The listing builds one solid part. Answer for the finished solid, in the listing's coordinates (mm). Face numbers are marked on the shaded views. A direction names the side the tool comes from. Give positions to 0.01 mm unless a question says otherwise; leave off trailing zeros. Loops run counter-clockwise (first coordinate to the right, second up) from the corner with the lowest first, then second, coordinate; pieces in that order, holes last. Notation, with made-up numbers: M 19,48.25 L 24,48.25 A17 ccw 24,69.25 Z; hole C 38.5,73 d7. An arc over 180 degrees is marked long. Use one line per item in the form item = value. Start each with the question number.
1. The mould has two halves that part along X. Classify the marked faces 1, 2 and 3: released by +X, released by -X, zero draft, split by the parting line, or undercut.
2. The part is cut by section C-C (z = 5). Write down the section's boundary in (x, y).
3. Straight lines are drawn through the part: line 1 (Y direction, x = 0, z = 7); line 2 (Z direction, x = 3, y = -2.75); line 3 (X direction, y = 1.25, z = 8.25). For each, find the intervals that lie inside material, in ascending order. Write a range as from..to.
4. For the marked faces 4 and 5, determine the directions among +Z, -Z, +X, -X, +Y, -Y from which every point of the face is accessible in a straight line to the end or side of a thin tool.
5. The part is cut by section A-A (y = 0). Write down the section's boundary in (x, z).
6. Each of these flat-tipped pins is pushed along its axis until it touches: pin 1 Ø3.5 at (x, y) = (0, 0) entering from -Z; pin 2 Ø4 at (x, z) = (-1.5, 6) entering from -Y. Where does it stop, or does it pass through?
Autodesk Inventor part; units mm, degrees
ref_plane "YZ Plane" through (0, 0, 0) normal (1, 0, 0) x (0, 1, 0)
ref_plane "XZ Plane" through (0, 0, 0) normal (0, 1, 0) x (-1, 0, 0)
ref_plane "XY Plane" through (0, 0, 0) normal (0, 0, 1) x (1, 0, 0)
sketch "Skizze1" plane through (0, 0, 0) normal (0, 0, 1) x (1, 0, 0)
  line L0 (-2.15, 4.15) -> (2.15, 4.15)
  line L1 (4.15, 2.15) -> (4.15, -2.15)
  line L2 (2.15, -4.15) -> (-2.15, -4.15)
  line L3 (-4.15, -2.15) -> (-4.15, 2.15)
  arc A0 (-2.15, 4.15) -> (-4.15, 2.15) centre (-2.15, 2.15) ccw
  arc A1 (4.15, 2.15) -> (2.15, 4.15) centre (2.15, 2.15) ccw
  arc A2 (2.15, -4.15) -> (4.15, -2.15) centre (2.15, -2.15) ccw
  arc A3 (-4.15, -2.15) -> (-2.15, -4.15) centre (-2.15, -2.15) ccw
  line L4 (-2.15, 2.15) -> (2.15, -2.15) construction
  line L5 (2.15, 2.15) -> (-2.15, -2.15) construction
  point P0 (0, 0)
  dimension "d0" = 2
  dimension "d1" = 8.3
extrude "Extrusion1" add sketch "Skizze1" along normal blind 3
sketch "Skizze2" plane through (0, 0, 3) normal (0, 0, 1) x (1, 0, 0)
  circle A0 centre (0, 0) radius 4
  dimension "d4" = 8
extrude "Extrusion2" add sketch "Skizze2" along normal blind 12
thread "Gewinde1"
sketch "Skizze3" plane through (0, 0, 15) normal (0, 0, 1) x (1, 0, 0)
  point P0 (0, 0)
  point P1 (0, 0)
hole "Bohrung1" at (0, 0, 15) direction (0, 0, -1) diameter 4 end through all
chamfer "Fase1" distance 1 angle 45 1 edges at (-4, 0, 15)
properties part number "Radadapter" material "Aluminium 6061"
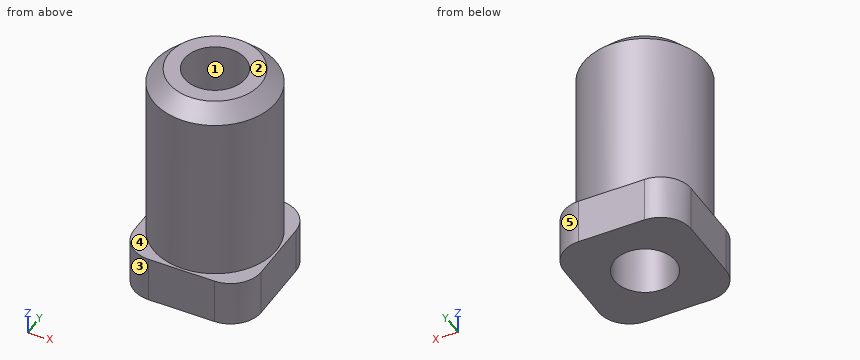
Derived:
q1.face_1 = undercut
q1.face_2 = zero draft
q1.face_3 = released by -X
q2.outline = C 0,0 d8; hole C 0,0 d4
q3.line_1 = -4..-2, 2..4
q3.line_2 = 0..3
q3.line_3 = -3.8..-1.56, 1.56..3.8
q4.face_4 = +Z
q4.face_5 = +Z, -Z, +X, +Y
q5.outline = M -4.15,0 L -2,0 L -2,15 L -3,15 L -4,14 L -4,3 L -4.15,3 Z; M 2,0 L 4.15,0 L 4.15,3 L 4,3 L 4,14 L 3,15 L 2,15 Z
q6.pin_1 = through
q6.pin_2 = -4
